from build123d import *

# Parameters (mm, degrees)
BOSS_EXTRUDE1_DEPTH = 150
SKETCH3_W           = 35
SKETCH3_H           = 80
CUT_EXTRUDE1_DEPTH  = 150
SKETCH5_W           = 7.5
SKETCH5_H           = 9.5
CUT_EXTRUDE3_DEPTH  = 7
SKETCH6_W           = 7.5
SKETCH6_H           = 9
CUT_EXTRUDE4_DEPTH  = 5
SKETCH7_W           = 66.039270253
SKETCH7_H           = 79.533085961
CUT_EXTRUDE5_DEPTH  = 70


with BuildPart() as part:
    # Sketch2 → Boss-Extrude1 (new body)
    with BuildSketch(Plane.XY):
        with BuildLine():
            Line((0, 0), (-35, 0))
            Line((-35, 0), (-35, 19))
            Line((-35, 19), (-9, 45))
            Line((-9, 45), (0, 45))
            Line((0, 45), (0, 25.5))
            ThreePointArc((0, 25.5), (-12.5, 13), (0, 0.5))
            Line((0, 0.5), (0, 0))
        make_face()
    extrude(amount=BOSS_EXTRUDE1_DEPTH)

    # Sketch3 → Cut-Extrude1 (cut)
    with BuildSketch(Plane.XZ):
        with Locations((-17.5, 75)):
            Rectangle(SKETCH3_W, SKETCH3_H)
    extrude(amount=-CUT_EXTRUDE1_DEPTH, mode=Mode.SUBTRACT)


with BuildPart() as cut_extrude1_piece_1:
    # of the separate pieces the step leaves, piece 1, a body of its own (cut_extrude1_pieces)
    add(part.part.solids().sort_by_distance((0, 0.5, 115))[0])


with BuildPart() as cut_extrude1_piece_2:
    # of the separate pieces the step leaves, piece 2, a body of its own (cut_extrude1_pieces)
    add(part.part.solids().sort_by_distance((0, 25.5, 0))[0])


with BuildPart() as cut_extrude3_tool:
    # Sketch5 → Cut-Extrude3 (new body)
    with BuildSketch(Plane(origin=(0, 0, 0), x_dir=(0, 0, -1), z_dir=(1, 0, 0))):
        with Locations((-118.75, 35.25)):
            Rectangle(SKETCH5_W, SKETCH5_H)
        with Locations((-31.25, 35.25)):
            Rectangle(SKETCH5_W, SKETCH5_H)
    extrude(amount=-CUT_EXTRUDE3_DEPTH)


with BuildPart() as cut_extrude1_piece_1_1:
    add(cut_extrude1_piece_1.part)

    # Cut-Extrude3: cut by cut_extrude3_tool
    add(cut_extrude3_tool.part, mode=Mode.SUBTRACT)


with BuildPart() as cut_extrude1_piece_2_1:
    add(cut_extrude1_piece_2.part)

    # Cut-Extrude3: cut by cut_extrude3_tool
    add(cut_extrude3_tool.part, mode=Mode.SUBTRACT)


with BuildPart() as cut_extrude4_tool:
    # Sketch6 → Cut-Extrude4 (new body)
    with BuildSketch(Plane.ZY.offset(35)):
        with Locations((31.25, 9.5)):
            Rectangle(SKETCH6_W, SKETCH6_H)
        with Locations((118.75, 9.5)):
            Rectangle(SKETCH6_W, SKETCH6_H)
    extrude(amount=-CUT_EXTRUDE4_DEPTH)


with BuildPart() as cut_extrude1_piece_1_2:
    add(cut_extrude1_piece_1_1.part)

    # Cut-Extrude4: cut by cut_extrude4_tool
    add(cut_extrude4_tool.part, mode=Mode.SUBTRACT)

    # Sketch7 → Cut-Extrude5 (cut)
    with BuildSketch(Plane.ZY.offset(35)):
        with Locations((129.10930736, 20.534013606)):
            Rectangle(SKETCH7_W, SKETCH7_H)
    extrude(amount=-CUT_EXTRUDE5_DEPTH, mode=Mode.SUBTRACT)


with BuildPart() as cut_extrude1_piece_2_2:
    add(cut_extrude1_piece_2_1.part)

    # Cut-Extrude4: cut by cut_extrude4_tool
    add(cut_extrude4_tool.part, mode=Mode.SUBTRACT)


solid = cut_extrude1_piece_2_2.part
Verification items for the finished model (mm, model axes). A direction names the side the tool comes from. Coordinates: 2 decimals unless noted, no trailing zeros. Loops run counter-clockwise (first coordinate to the right, second up) from the corner with the lowest first, then second, coordinate; pieces in that order, holes last. Notation, with made-up numbers: (42, -24) -> (50, -24) arc R22 cw to (50, -3) -> close; hole circle Ø9 at (64, -25.5). An arc over 180 degrees is marked (long way). Write each question's results on one line, items separated by ' | '.
Item 1: Section check A-A, the plane x = -3.5. Enter the section's corners in (y, z), plus the area to 3 significant figures.
Found:
outline: (0, 0) -> (1, 0) -> (1, 35) -> (0, 35) -> close; (25, 0) -> (45, 0) -> (45, 35) -> (40, 35) -> (40, 27.5) -> (30.5, 27.5) -> (30.5, 35) -> (25, 35) -> close | area: 664 mm2
Item 2: Section check D-D, the plane x = -31. Enter the section's corners in (y, z).
Found:
outline: (0, 0) -> (23, 0) -> (23, 35) -> (14, 35) -> (14, 27.5) -> (5, 27.5) -> (5, 35) -> (0, 35) -> close
Item 3: Section check C-C, the plane y = 13. Enter the section's corners in (x, z).
Found:
outline: (-35, 0) -> (-12.5, 0) -> (-12.5, 35) -> (-30, 35) -> (-30, 27.5) -> (-35, 27.5) -> close
Item 4: Gauge pin test, flat ends, axial feed: pin 1 (5 mm diameter, centred on y = 20, z = 13.5, fed in from +X); pin 2 (6 mm diameter, centred on y = 34.5, z = 32.5, fed in from +X); pin 3 (5.5 mm diameter, centred on x = -2, y = 36.5, fed in from +Z). Record the tip position at first contact, or that the pin passes through.
Found:
pin 1: stops at x = -8.12 | pin 2: stops at x = -7 | pin 3: stops at z = 27.5
Item 5: Mould release check, pull along Y, two halves, no side actions. Record for faces 1 (the face through (-17, 0, 17)), 2 (the face through (-33, 14, 31)), 3 (the face through (-17, 23, 0)): +Y half, -Y half, draft (parallel to the pull), parting line (faces both ways), or undercut.
Found:
face 1: -Y half | face 2: undercut | face 3: draft
Item 6: Section check B-B, the plane z = 6.5. Enter the section's corners in (x, y).
Found:
outline: (-35, 0) -> (0, 0) -> (0, 0.5) arc R12.5 cw to (0, 25.5) -> (0, 45) -> (-9, 45) -> (-35, 19) -> close
Item 7: Material ranges on L1, parallel to Y at x = -4, z = 33.5; L2, parallel to Y at x = -20, z = 8.5; L3, parallel to X at y = 24.5, z = 29, recorded low to high.
Found:
L1: y = 0 to 1.16, 24.84 to 30.5, 40 to 45 | L2: y = 0 to 34 | L3: x = -29.5 to -4.9
Item 8: Tool access check on faces 4 (the face through (-3, 40, 31)), 5 (the face through (0, 35, 17)), 6 (the face through (-33, 9, 27.5)). Record the directions out of +Z, -Z, +X, -X, +Y, -Y that give a thin tool (end or side, any length) a straight path to the whole face; none if there is none.
Found:
face 4: +Z, +X | face 5: +Z, -Z, +X, +Y, -Y | face 6: +Z, -X
